```python
from build123d import *

# Parameters (mm, degrees)
F0_R     = 29.322045
F1_DEPTH = 3
F2_R     = 27.665962
F3_DEPTH = 1.5
F4_R     = 6.073968
F5_DEPTH = 3
F7_D     = 4
F7_DEPTH = 2


with BuildPart() as f1:
    # F0 (on Top) → F1 (new body)
    with BuildSketch(Plane.XY):
        Circle(F0_R)
    extrude(amount=F1_DEPTH)

    # F2 (on face) → F3 (cut)
    with BuildSketch(Plane.XY.offset(3)):
        Circle(F2_R)
    extrude(amount=-F3_DEPTH, mode=Mode.SUBTRACT)

    # F4 (on face) → F5 (join)
    with BuildSketch(Plane.XY.offset(1.5)):
        Circle(F4_R)
        with BuildLine():
            ThreePointArc((-11.182132, 22.020222), (-21.055439, 12.909818), (-24.772728, 0))
            Line((-24.772728, 0), (-9.090909, 0))
            ThreePointArc((-9.090909, 0), (-7.576474, 4.79996), (-3.711611, 8.024237))
            Line((-3.711611, 8.024237), (-11.182132, 22.020222))
        make_face()
        with BuildLine():
            ThreePointArc((4.580156, 7.562137), (7.763511, 4.374334), (8.841026, 0))
            Line((8.841026, 0), (24.696766, 0))
            ThreePointArc((24.696766, 0), (21.471368, 12.52034), (12.163349, 21.493795))
            Line((12.163349, 21.493795), (4.580156, 7.562137))
        make_face()
        with BuildLine():
            ThreePointArc((-11.447483, -21.88345), (0.709798, -24.657945), (12.687344, -21.188694))
            Line((12.687344, -21.188694), (5.195707, -7.153148))
            ThreePointArc((5.195707, -7.153148), (0.777582, -8.821586), (-3.86429, -7.951793))
            Line((-3.86429, -7.951793), (-11.447483, -21.88345))
        make_face()
    extrude(amount=F5_DEPTH)

    # F7
    with Locations(Plane.XY.offset(1.5)):
        with Locations((0, 24.204547)):
            Hole(F7_D / 2, depth=F7_DEPTH)


solid = f1.part
```
Could you check a few things on this model? Use its own coordinates, in mm. A direction names the side the tool comes from. Round coordinates to 2 decimals unless told otherwise and drop trailing zeros. Loops run counter-clockwise (first coordinate to the right, second up) from the corner with the lowest first, then second, coordinate; pieces in that order, holes last.
Q1. I want a section at B-B (y = -13). Write out the boundary of the cut face in (x, z), and give its area (3 significant figures).
Q2. I want a section at D-D (y = 1). Write out the boundary of the cut face in (x, z), and give its area (3 significant figures).
Q3. Please list where these lines run through material, in increasing order: L1, parallel to Y at x = 0, z = 2.4; L2, parallel to X at y = 7, z = 2.3; L3, parallel to X at y = 3.5, z = 4.25.
Q4. I want a section at A-A (x = 0). Write out the boundary of the cut face in (y, z).
Q5. On a 3-axis mill with a long thin cutter (end or side, diameter ignored), from which of +Z, -Z, +X, -X, +Y, -Y can I reach the whole of each face in a straight line? I mean faces 4 (the cylindrical face through (21.563, 12.362, 2.979)), 5 (the flat face through (15, 9, 4.5)). Say none if no direction works.
Q6. Thinking about a two-plate mould opening in X: for faces 1 (the cylindrical face through (-6.356, -28.625, 1.479)), 2 (the flat face through (0, 0, 4.5)), 3 (the cylindrical face through (7.73, 4.43, 2.98)), which applies, pulls with the +X half, pulls with the -X half, needs draft (parallel to the pull), parting line crosses it, or undercut?
Q7. I want a section at C-C (x = 25.5). Write out the boundary of the cut face in (y, z), and give its area (3 significant figures).
Q8. For P1, Ø1, axis at y = 18.5, z = 2, coming from the +X side; P2, Ø2.5, axis at x = -16, z = 3.5, coming from the -Y side; P3, Ø6, axis at x = 16, y = -22, coming from the +Z side, each with a flat end and sliding along its axis, tell me the tip position at first contact or that it passes through.
Answer below:
1. outline: (-26.28, 0) - (26.28, 0) - (26.28, 3) - (24.42, 3) - (24.42, 1.5) - (8.32, 1.5) - (8.32, 4.5) - (-6.61, 4.5) - (-6.61, 1.5) - (-24.42, 1.5) - (-24.42, 3) - (-26.28, 3) - close
1. area: 129 mm2
2. outline: (-29.3, 0) - (29.3, 0) - (29.3, 3) - (27.65, 3) - (27.65, 1.5) - (24.7, 1.5) - (24.7, 4.5) - (8.81, 4.5) - (8.81, 1.5) - (5.99, 1.5) - (5.99, 4.5) - (-5.99, 4.5) - (-5.99, 1.5) - (-9.01, 1.5) - (-9.01, 4.5) - (-24.74, 4.5) - (-24.74, 1.5) - (-27.65, 1.5) - (-27.65, 3) - (-29.3, 3) - close
2. area: 224 mm2
3. L1: y = -29.32 to -27.67, -24.67 to -8.86, -6.07 to 6.07, 27.67 to 29.32
3. L2: x = -28.47 to -26.77, -23.71 to -5.48, 5.45 to 23.81, 26.77 to 28.47
3. L3: x = -24.5 to -8.3, -4.96 to 4.96, 8.19 to 24.52
4. outline: (-29.32, 0) - (22.2, 0) - (22.2, 1.5) - (6.07, 1.5) - (6.07, 4.5) - (-6.07, 4.5) - (-6.07, 1.5) - (-8.86, 1.5) - (-8.86, 4.5) - (-24.67, 4.5) - (-24.67, 1.5) - (-27.67, 1.5) - (-27.67, 3) - (-29.32, 3) - close; (26.2, 0) - (29.32, 0) - (29.32, 3) - (27.67, 3) - (27.67, 1.5) - (26.2, 1.5) - close
5. face 4: +Z
5. face 5: +Z, +X, -X, +Y, -Y
6. face 1: parting line crosses it
6. face 2: needs draft
6. face 3: undercut
7. outline: (-14.48, 0) - (14.48, 0) - (14.48, 3) - (10.73, 3) - (10.73, 1.5) - (-10.73, 1.5) - (-10.73, 3) - (-14.48, 3) - close
7. area: 54.7 mm2
8. P1: stops at x = 23.15
8. P2: stops at y = -25.28
8. P3: stops at z = 3
